Here's the drawing with two shaded views (mm, measured from the low corner). I have some questions. A direction names the side the tool comes from. Coordinates: 2 decimals unless noted, no trailing zeros. Order: outer loops, then holes, each group sorted by start corner. A loop starts at its lowest first (then second) coordinate and runs counter-clockwise, first axis right, second up. Notation, with made-up numbers: (46.25, 65) - (91.25, 65) arc R21 cw to (91.25, 104) - close; hole circle Ø9 at (-35.5, 63.25). An arc over 180 degrees is marked (long way). Answer as a JSON object with one key per item and string values. Group by question number.
(1) Which directions (+Z, -Z, +X, -X, +Y, -Y) give clear straight access to the entire face, cutting with the end or side of a thin tool? Please do the marked faces 1 and 2.
(2) Imagine slicing it at A-A, the plane y = 8. Write out the boundary of the cut face in (x, z), and give its area (3 significant figures).
(3) Imagine slicing it at D-D, the plane z = 6.5. Write out the boundary of the cut face in (x, y).
(4) We'd pull the mould along X, two halves only. Please class the marked faces 3, 4 and 5: pulls with the +X half, pulls with the -X half, needs draft (parallel to the pull), parting line crosses it, or undercut.
(5) Imagine slicing it at C-C, the plane y = 30.5. Write out the boundary of the cut face in (x, z), and give its area (3 significant figures).
(6) Please list where these lines run through material, in increasing order: probe 1 along X at (y, z) = (5, 16); probe 2 along Y at (x, z) = (21.25, 10); probe 3 along Y at (x, z) = (5, 30.55).
(7) Will this pin go through, and if not, where does the flat tip stop? P1, Ø7, axis at x = 16.5, y = 11.5, coming from the -Z side.
(8) Imagine slicing it at B-B, the plane x = 5. Write out the boundary of the cut face in (y, z), and give its area (3 significant figures).
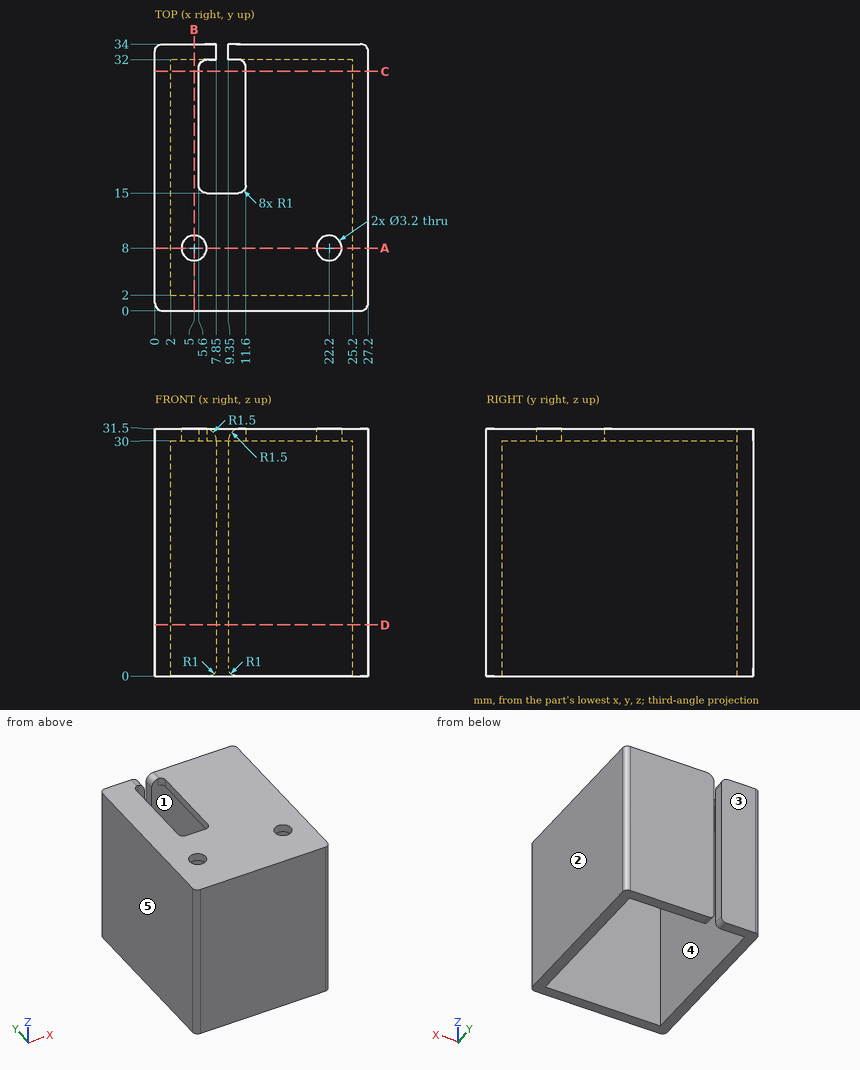
Result set:
{
 "1": {"face 1": "-Z", "face 2": "+Z, -Z, +X, +Y, -Y"},
 "2": {"outline": "(0, 0) - (2, 0) - (2, 30) - (3.4, 30) - (3.4, 31.5) - (0, 31.5) - close; (6.6, 30) - (20.6, 30) - (20.6, 31.5) - (6.6, 31.5) - close; (23.8, 30) - (25.2, 30) - (25.2, 0) - (27.2, 0) - (27.2, 31.5) - (23.8, 31.5) - close", "area": "151 mm^2"},
 "3": {"outline": "(0, 1) arc R1 ccw to (1, 0) - (26.2, 0) arc R1 ccw to (27.2, 1) - (27.2, 33) arc R1 ccw to (26.2, 34) - (9.35, 34) - (9.35, 32) - (25.2, 32) - (25.2, 2) - (2, 2) - (2, 32) - (7.85, 32) - (7.85, 34) - (1, 34) arc R1 ccw to (0, 33) - close"},
 "4": {"face 3": "needs draft", "face 4": "undercut", "face 5": "pulls with the -X half"},
 "5": {"outline": "(0, 0) - (2, 0) - (2, 30) - (5.6, 30) - (5.6, 31.5) - (0, 31.5) - close; (11.6, 30) - (25.2, 30) - (25.2, 0) - (27.2, 0) - (27.2, 31.5) - (11.6, 31.5) - close", "area": "152 mm^2"},
 "6": {"probe 1": "x = 0 to 2, 25.2 to 27.2", "probe 2": "y = 0 to 2, 32 to 34", "probe 3": "y = 0 to 6.4, 9.6 to 34"},
 "7": {"P1": "stops at z = 30"},
 "8": {"outline": "(0, 0) - (2, 0) - (2, 30) - (6.4, 30) - (6.4, 31.5) - (0, 31.5) - close; (9.6, 30) - (32, 30) - (32, 0) - (34, 0) - (34, 31.5) - (9.6, 31.5) - close", "area": "166 mm^2"}
}
